from build123d import *

# Parameters (mm, degrees)
ESQUISSE1_R             = 10.3
BOSS_EXTRU_1_DEPTH      = 2.1
ESQUISSE2_R             = 4.8
BOSS_EXTRU_2_DEPTH      = 3.3
ESQUISSE3_R             = 1.65
ENL_V_MAT_EXTRU_1_DEPTH = 16.535121499


with BuildPart() as part:
    # Esquisse1 → Boss.-Extru.1 (new body)
    with BuildSketch(Plane.XY):
        Circle(ESQUISSE1_R)
    extrude(amount=BOSS_EXTRU_1_DEPTH)

    # Esquisse2 → Boss.-Extru.2 (add)
    with BuildSketch(Plane.XY):
        Circle(ESQUISSE2_R)
    extrude(amount=-BOSS_EXTRU_2_DEPTH)

    # Esquisse3 → Enlèv. mat.-Extru.1 (cut, through all)
    with BuildSketch(Plane.XY.offset(2.1)):
        with Locations((7.95, 0)):
            Circle(ESQUISSE3_R)
        with Locations((-7.95, 0)):
            Circle(ESQUISSE3_R)
    extrude(amount=-ENL_V_MAT_EXTRU_1_DEPTH, mode=Mode.SUBTRACT)

    # Esquisse4 → Chambrage pour vis à six pans creux M31 (revolve, cut)
    with BuildSketch(Plane(origin=(0, 0, 2.1), x_dir=(0, -1, 0), z_dir=(1, 0, 0))):
        Polygon((0, 0), (0, 5.4), (1.7, 5.4), (1.7, 3.4), (3.25, 3.4), (3.25, 0), align=None)
    revolve(axis=Axis((0, 0, 8.45), (0, 0, -1)), mode=Mode.SUBTRACT)


solid = part.part
Could you check a few things on this model? Use its own coordinates, in mm. A direction names the side the tool comes from. Give positions to 0.01 mm unless a question says otherwise; leave off trailing zeros. Loops run counter-clockwise (first coordinate to the right, second up) from the corner with the lowest first, then second, coordinate; pieces in that order, holes last. Notation, with made-up numbers: (34.25, 74) -> (45.25, 74) arc R30 ccw to (45.25, 109) -> close; hole circle Ø4 at (6, -32). An arc over 180 degrees is marked (long way). Return JSON: item names as keys, results as strings.
Item 1: If we section it at C-C on z = -2.4: List the corners of the cut face in (x, y) for me, plus the area to 3 significant figures.
Geometry results:
{"outline": "circle Ø9.6 at (0, 0); hole circle Ø3.4 at (0, 0)", "area": "63.3 mm²"}
Item 2: If we section it at A-A on y = 0: List the corners of the cut face in (x, z) for me.
Geometry results:
{"outline": "(-10.3, 0) -> (-9.6, 0) -> (-9.6, 2.1) -> (-10.3, 2.1) -> close; (-6.3, 0) -> (-4.8, 0) -> (-4.8, -3.3) -> (-1.7, -3.3) -> (-1.7, -1.3) -> (-3.25, -1.3) -> (-3.25, 2.1) -> (-6.3, 2.1) -> close; (1.7, -3.3) -> (4.8, -3.3) -> (4.8, 0) -> (6.3, 0) -> (6.3, 2.1) -> (3.25, 2.1) -> (3.25, -1.3) -> (1.7, -1.3) -> close; (9.6, 0) -> (10.3, 0) -> (10.3, 2.1) -> (9.6, 2.1) -> close"}
Item 3: If we section it at B-B on x = 0: List the corners of the cut face in (y, z) for me.
Geometry results:
{"outline": "(-10.3, 0) -> (-4.8, 0) -> (-4.8, -3.3) -> (-1.7, -3.3) -> (-1.7, -1.3) -> (-3.25, -1.3) -> (-3.25, 2.1) -> (-10.3, 2.1) -> close; (1.7, -3.3) -> (4.8, -3.3) -> (4.8, 0) -> (10.3, 0) -> (10.3, 2.1) -> (3.25, 2.1) -> (3.25, -1.3) -> (1.7, -1.3) -> close"}
Item 4: Which directions (+Z, -Z, +X, -X, +Y, -Y) give clear straight access to the entire face, cutting with the end or side of a thin tool? Please do faces 1 (the flat face through (-2.43, 2.43, 2.1)), 2 (the cylindrical face through (1.978, 2.579, 0.424)), 3 (the flat face through (4.4, 2.4, 0)).
Geometry results:
{"face 1": "+Z, +X, -X, +Y, -Y", "face 2": "+Z", "face 3": "-Z"}
Item 5: I'm going to push flat-ended pins straight in: pin 1 (6 mm diameter, centred on x = 5, y = 6.5, fed in from -Z); pin 2 (1 mm diameter, centred on y = -7.5, z = 0.5, fed in from -X); pin 3 (2 mm diameter, centred on x = -7.5, z = -0.5, fed in from +Y). Where does each tip first touch, or does it pass through?
Geometry results:
{"pin 1": "stops at z = 0", "pin 2": "stops at x = -7.56", "pin 3": "stops at y = 7.88"}
Item 6: If we section it at D-D on y = -2.25: List the corners of the cut face in (x, z) for me.
Geometry results:
{"outline": "(-10.05, 0) -> (-4.24, 0) -> (-4.24, -3.3) -> (4.24, -3.3) -> (4.24, 0) -> (10.05, 0) -> (10.05, 2.1) -> (2.35, 2.1) -> (2.35, -1.3) -> (-2.35, -1.3) -> (-2.35, 2.1) -> (-10.05, 2.1) -> close"}
Item 7: We'd pull the mould along Y, two halves only. Please class faces 4 (the cylindrical face through (-6.376, 0.496, 1.065)), 5 (the flat face through (2, 0, -3.3)), 6 (the cylindrical face through (2.58, 4.05, -1.63)), 7 (the flat face through (1.4, 1.4, -1.3)): +Y half, -Y half, draft (parallel to the pull), parting line (faces both ways), or undercut.
Geometry results:
{"face 4": "undercut", "face 5": "draft", "face 6": "parting line", "face 7": "undercut"}
Item 8: I need wall thicknesses on L1, parallel to Y at x = 0, z = -0.6; L2, parallel to X at y = -2, z = 0.1; L3, parallel to Y at x = -7.95, z = 0.7. Which ranges of each line are inside material? Lowest first, please. Write a range as from..to.
Geometry results:
{"L1": "y = -4.8..-3.25, 3.25..4.8", "L2": "x = -10.1..-2.56, 2.56..10.1", "L3": "y = -6.55..-1.65, 1.65..6.55"}
